from build123d import *

# Parameters (mm, degrees)
F0_R     = 12.269655
F1_DEPTH = 46
F2_R     = 7.001219
F3_R     = 7.966905


with BuildPart() as f1:
    # F0 (on Right) → F1 (new body)
    with BuildSketch(Plane.YZ):
        Circle(F0_R)
    extrude(amount=-F1_DEPTH)

    # F2
    f2_edges = [f1.edges().sort_by_distance(p)[0] for p in [
        (-46, -12.269655, 0),
    ]]
    fillet(f2_edges, radius=F2_R)

    # F3
    f3_edges = [f1.edges().sort_by_distance(p)[0] for p in [
        (0, -12.269655, 0),
    ]]
    fillet(f3_edges, radius=F3_R)


solid = f1.part
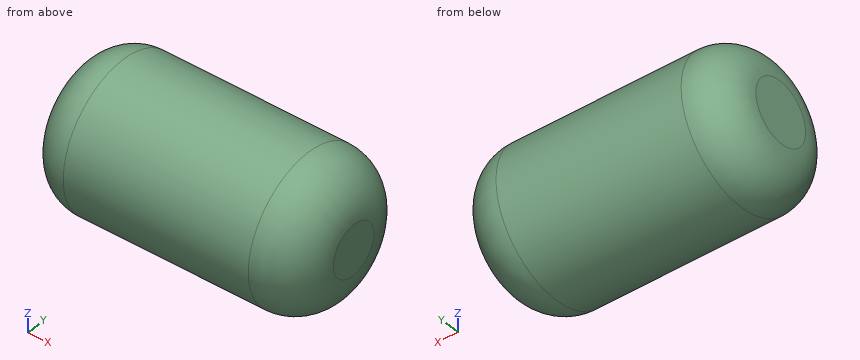
Geometry: final body of the model. Coordinates: model frame, mm. Coordinates: 2 decimals unless noted, no trailing zeros. Order: outer loops, then holes, each group sorted by start corner. A loop starts at its lowest first (then second) coordinate and runs counter-clockwise, first axis right, second up.
1) First-contact query: P1, Ø12, axis at x = -27, z = 8.5, coming from the +Y side; P2, Ø6, axis at y = -5.5, z = -9.5, coming from the -X side; P3, Ø4, axis at x = -37.5, z = 4.5, coming from the -Y side. Flat tips, straight axial feed; report the tip coordinate or a pass-through.
Result sheet:
P1: stops at y = 12.01
P2: stops at x = -45.45
P3: stops at y = -12.01
2) Ray query, probe 1 along Z at (x, y) = (-32, -0.5); probe 2 along X at (y, z) = (-3.75, -3.5); probe 3 along Z at (x, y) = (-29, -3.5). Return the intervals inside material, ascending.
Result sheet:
probe 1: z = -12.26 to 12.26
probe 2: x = -46 to -0.04
probe 3: z = -11.76 to 11.76
3) Section A-A (x = -29.5). Return loops of the section in (y, z).
Result sheet:
outline: circle Ø24.54 at (0, 0)
